Autodesk Inventor part; units mm, degrees
ref_plane "Work Plane2" through (0, 15.0876, -10.414) normal (0, 1, 0) x (-1, 0, 0)
ref_plane "YZ Plane" through (0, 0, 0) normal (1, 0, 0) x (0, 1, 0)
ref_plane "XZ Plane" through (0, 0, 0) normal (0, 1, 0) x (-1, 0, 0)
sketch "Sketch4" plane through (0, 0, 0) normal (0, 0, 1) x (1, 0, 0)
  circle A0 centre (0, 0) radius 18.923
  dimension "d2" = 37.846
extrude "Extrusion1" add sketch "Sketch4" against normal blind 10.414
sketch "Sketch7" plane through (0, 0, 0) normal (0, 0, 1) x (1, 0, 0)
  circle A0 centre (0, 0) radius 9.525
  dimension "d8" = 19.05
extrude "Extrusion3" cut sketch "Sketch7" against normal blind 127
sketch "Sketch8" plane through (0, 0, 0) normal (0, 0, 1) x (1, 0, 0)
  circle A0 centre (0, 0) radius 11.938
  dimension "d11" = 23.876
extrude "Extrusion4" cut sketch "Sketch8" against normal blind 3.9624
sketch "Sketch9" plane through (0, 0, -10.414) normal (0, 0, -1) x (-1, 0, 0)
  circle A0 centre (0, 0) radius 15.0876
  dimension "d14" = 30.1752
extrude "Extrusion5" add sketch "Sketch9" along normal blind 8.5852
sketch "Sketch10" plane through (0, 0, -10.414) normal (0, 0, 1) x (1, 0, 0)
  circle A0 centre (0, 0) radius 9.525
extrude "Extrusion6" cut sketch "Sketch10" against normal blind 8.5852
fillet "Fillet1" radius 1.6002 1 edges at (15.0876, 0, -10.414)
fillet "Fillet2" radius 1.6002 1 edges at (-18.923, 0, -10.414)
sketch "Sketch11" plane through (0, 0, -18.9992) normal (0, 0, -1) x (-1, 0, 0)
  circle A0 centre (0, 0) radius 9.525
  line L0 (0, 9.525) -> (0, 15.0876)
  circle A1 centre (0, 0) radius 15.0876
ref_plane "Work Plane2" through (0, 15.0876, -10.414) normal (0, 1, 0) x (-1, 0, 0)
sketch "Sketch12" plane through (0, 15.0876, -10.414) normal (0, 1, 0) x (-1, 0, 0)
  line L0 (0, 10.414) -> (0, -3.8354)
  dimension "d21" = 14.2494
hole "Hole1" at (0, 15.0876, -14.2494) direction (0, -1, 0) diameter 3.9624 depth 7.2644
fillet "Fillet3" radius 1.6002 1 edges at (15.0876, 0, -18.9992)
properties part number "Problem14_15_JacobMorgan_031015_pd3" material "Bronze"
The model under review builds one solid part; all positions refer to its coordinate system, in mm. A direction names the side the tool comes from. Round coordinates to 2 decimals unless told otherwise and drop trailing zeros. Loops run counter-clockwise (first coordinate to the right, second up) from the corner with the lowest first, then second, coordinate; pieces in that order, holes last. Notation, with made-up numbers: (-24.5, 73.25) -> (20.5, 73.25) arc R22 cw to (20.5, 105.25) -> close; hole circle Ø2 at (54, 87.25). An arc over 180 degrees is marked (long way). Write item = value, one per line. Start each with the question number.
Item 1: To check wall thickness, follow L1, parallel to Y at x = 0, z = -1.1; L2, parallel to Z at x = 0, y = 11.6; L3, parallel to Y at x = -5, z = -2.25. State the ranges of each line that lie inside material, in increasing order.
Item 2: Take a section at C-C on z = -7. Give the boundary of the cut face in (x, y) (3 decimals), plus the area to 3 significant figures.
Item 3: Mouldability with a two-part tool opening along Z and no side actions: class faces 4 (the flat face through (-1, -10, -3.962)), 5 (the cylindrical face through (18.05, 5.68, -4.35)), 6 (the cylindrical face through (-0.6, 12.16, -12.36)) as released by +Z, released by -Z, zero draft, split by the parting line, or undercut.
Item 4: Insertion check: pin 1 (12 mm diameter, centred on x = 1.5, y = -3.5, fed in from +Z); pin 2 (6 mm diameter, centred on x = -10, z = -16.5, fed in from +Y); pin 3 (2.5 mm diameter, centred on x = 0, z = -14.25, fed in from -Y); pin 4 (2 mm diameter, centred on x = 2, y = 7.5, fed in from -Z). Each pin has a flat end and moves straight along its axis. Give the tip position at first contact, or say it passes through.
Item 5: Take a section at A-A on y = 0. Give the boundary of the cut face in (x, z) (3 decimals), plus the area to 3 significant figures.
Item 6: Take a section at D-D on z = -12.75. Give the boundary of the cut face in (x, y) (3 decimals), plus the area to 3 significant figures.
Item 7: Take a section at B-B on x = 0. Give the boundary of the cut face in (y, z) (3 decimals).
Item 8: For faces 1 (the cylindrical face through (11.973, 9.181, -14.669)), 2 (the cylindrical face through (-2.06, -9.3, -11.38)), 3 (the cylindrical face through (-2.588, -11.654, -1.953)), list the 3-axis set-ups (+Z, -Z, +X, -X, +Y, -Y) from which the entire face can be reached by the end or side of a thin tool; tool diameter is ignored.
Result:
q1.L1 = -18.92 to -11.94, 11.94 to 18.92
q1.L2 = -19 to -16.23, -12.27 to -3.96
q1.L3 = -18.25 to -10.84, 10.84 to 18.25
q2.outline = circle Ø37.846 at (0, 0); hole circle Ø19.05 at (0, 0)
q2.area = 840 mm²
q3.face_4 = released by +Z
q3.face_5 = zero draft
q3.face_6 = undercut
q4.pin_1 = -3.96
q4.pin_2 = 13.37
q4.pin_3 = -15.09
q4.pin_4 = through
q5.outline = (-18.923, -8.814) arc R1.6 ccw to (-17.323, -10.414) -> (-16.688, -10.414) arc R1.6 cw to (-15.088, -12.014) -> (-15.088, -17.399) arc R1.6 ccw to (-13.487, -18.999) -> (-9.525, -18.999) -> (-9.525, -3.962) -> (-11.938, -3.962) -> (-11.938, 0) -> (-18.923, 0) -> close; (9.525, -18.999) -> (13.487, -18.999) arc R1.6 ccw to (15.088, -17.399) -> (15.088, -12.014) arc R1.6 cw to (16.688, -10.414) -> (17.323, -10.414) arc R1.6 ccw to (18.923, -8.814) -> (18.923, 0) -> (11.938, 0) -> (11.938, -3.962) -> (9.525, -3.962) -> close
q5.area = 271 mm²
q6.outline = (-1.295, 9.437) -> (-1.295, 15.032) arc R15.088 ccw (long way) to (1.295, 15.032) -> (1.295, 9.437) arc R9.525 cw (long way) to start
q6.area = 416 mm²
q7.outline = (-18.923, -8.814) arc R1.6 ccw to (-17.323, -10.414) -> (-16.688, -10.414) arc R1.6 cw to (-15.088, -12.014) -> (-15.088, -17.399) arc R1.6 ccw to (-13.487, -18.999) -> (-9.525, -18.999) -> (-9.525, -3.962) -> (-11.938, -3.962) -> (-11.938, 0) -> (-18.923, 0) -> close; (9.525, -18.999) -> (13.487, -18.999) arc R1.6 ccw to (15.088, -17.399) -> (15.088, -16.231) -> (9.525, -16.231) -> close; (9.525, -12.268) -> (15.088, -12.268) -> (15.088, -12.014) arc R1.6 cw to (16.688, -10.414) -> (17.323, -10.414) arc R1.6 ccw to (18.923, -8.814) -> (18.923, 0) -> (11.938, 0) -> (11.938, -3.962) -> (9.525, -3.962) -> close
q8.face_1 = -Z
q8.face_2 = +Z, -Z
q8.face_3 = +Z
